Read the model definition and answer for the solid it produces. Units are mm, in the model's axes. A direction names the side the tool comes from. Coordinates: 2 decimals unless noted, no trailing zeros. Write each loop counter-clockwise with the first axis right and the second up, starting at its lowest first coordinate (ties: lowest second). Pieces come first, ordered by that corner, then holes. Notation, with made-up numbers: M -10,76 L 1,76 A23 cw 1,91 Z; hole C 47.25,15 d7. An arc over 180 degrees is marked long. Use a Markdown table: item, result. Add a question column.
from build123d import *

# Parameters (mm, degrees)
SKETCH1_W                                           = 75
SKETCH1_H                                           = 75
BOSS_EXTRUDE1_DEPTH                                 = 15
SKETCH2_R                                           = 22
BOSS_EXTRUDE2_DEPTH                                 = 5
CBORE_FOR_M5_HEX_SOCKET_HEAD_CAP_SCREW1_D           = 5.5
CBORE_FOR_M5_HEX_SOCKET_HEAD_CAP_SCREW1_CBORE_D     = 10
CBORE_FOR_M5_HEX_SOCKET_HEAD_CAP_SCREW1_CBORE_DEPTH = 5.4
CIRPATTERN1_COUNT                                   = 4
CHAMFER1_SIZE                                       = 6
SHELL1_START                                        = 3
SHELL1_OUTLINE_R                                    = 25
SHELL1_DEPTH                                        = 116.5
SHELL1_START_2                                      = -5
SHELL1_2_OUTLINE_R                                  = 14.94492882
SHELL1_2_DEPTH                                      = 206.012430393
SHELL1_3_OUTLINE_R                                  = 18.5
SHELL1_3_OUTLINE_R_2                                = 14.94492882
SHELL1_3_DEPTH                                      = 169.882661511
SHELL1_4_OUTLINE_R                                  = 25
SHELL1_4_DEPTH                                      = 9
SHELL1_5_OUTLINE_R                                  = 5.75
SHELL1_5_DEPTH                                      = 3.6
SHELL1_6_OUTLINE_R                                  = 19
SHELL1_6_OUTLINE_R_2                                = 18.5
SHELL1_6_DEPTH                                      = 8


with BuildPart() as part:
    # Sketch1 → Boss-Extrude1 (new body)
    with BuildSketch(Plane.XY):
        Rectangle(SKETCH1_W, SKETCH1_H)
    extrude(amount=BOSS_EXTRUDE1_DEPTH)

    # Sketch2 → Boss-Extrude2 (add)
    with BuildSketch(Plane(origin=(0, 0, 0), x_dir=(-1, 0, 0), z_dir=(0, 0, -1))):
        Circle(SKETCH2_R)
    extrude(amount=BOSS_EXTRUDE2_DEPTH)

    # Sketch3 → Revolve1 (revolve)
    with BuildSketch(Plane(origin=(0, 0, 0), x_dir=(0, 0, -1), z_dir=(1, 0, 0)), mode=Mode.PRIVATE) as revolve1_sk:
        Polygon((-15, 28), (-122.5, 28), (-122.5, 21.5), (-167.882661511, 21.5), (-167.882661511, 17.94492882), (-202.25507118, 17.94492882), (-207.2, 13), (-207.2, 0), (-15, 0), align=None)
    revolve(revolve1_sk.sketch.rotate(Axis((0, 0, 207.2), (0, 0, -1)), 90), axis=Axis((0, 0, 207.2), (0, 0, -1)))

    # CBORE for M5 Hex Socket Head Cap Screw1 (through all)
    with Locations(Plane.XY.offset(15)):
        with Locations((-27.5, 27.5)):
            cbore_for_m5_hex_socket_head_cap_screw1 = CounterBoreHole(CBORE_FOR_M5_HEX_SOCKET_HEAD_CAP_SCREW1_D / 2, CBORE_FOR_M5_HEX_SOCKET_HEAD_CAP_SCREW1_CBORE_D / 2, CBORE_FOR_M5_HEX_SOCKET_HEAD_CAP_SCREW1_CBORE_DEPTH)

    # CirPattern1: CBORE for M5 Hex Socket Head Cap Screw1 ×4 about axis
    cirpattern1_axis = Axis((0, 0, 0), (0, 0, 1))
    for i in range(1, CIRPATTERN1_COUNT):
        add(cbore_for_m5_hex_socket_head_cap_screw1.rotate(cirpattern1_axis, i * 360 / CIRPATTERN1_COUNT), mode=Mode.SUBTRACT)

    # Chamfer1
    chamfer1_edges = [part.edges().sort_by_distance(p)[0] for p in [
        (37.5, -37.5, 7.5),
        (-37.5, -37.5, 7.5),
        (-37.5, 37.5, 7.5),
        (37.5, 37.5, 7.5),
    ]]
    chamfer(chamfer1_edges, length=CHAMFER1_SIZE)

    # Shell1: read off the stored shape, not the designer's step
    # Shell1 outline → Shell1 (cut)
    with BuildSketch(Plane.XY.offset(SHELL1_START)):
        Circle(SHELL1_OUTLINE_R)
    extrude(amount=SHELL1_DEPTH, mode=Mode.SUBTRACT)

    # Shell1 2 outline → Shell1 2 (cut)
    with BuildSketch(Plane.XY.offset(SHELL1_START_2)):
        Circle(SHELL1_2_OUTLINE_R)
    extrude(amount=SHELL1_2_DEPTH, mode=Mode.SUBTRACT)

    # Shell1 3 outline → Shell1 3 (cut)
    with BuildSketch(Plane.XY.offset(SHELL1_START_2)):
        Circle(SHELL1_3_OUTLINE_R)
        Circle(SHELL1_3_OUTLINE_R_2, mode=Mode.SUBTRACT)
    extrude(amount=SHELL1_3_DEPTH, mode=Mode.SUBTRACT)

    # Shell1 4 outline → Shell1 4 (cut)
    with BuildSketch(Plane.XY.offset(SHELL1_START)):
        with BuildLine():
            Line((-34.5, 23.627016654), (-34.5, -23.627016654))
            ThreePointArc((-34.5, -23.627016654), (-21.843145751, -21.843145751), (-23.627016654, -34.5))
            Line((-23.627016654, -34.5), (23.627016654, -34.5))
            ThreePointArc((23.627016654, -34.5), (21.843145751, -21.843145751), (34.5, -23.627016654))
            Line((34.5, -23.627016654), (34.5, 23.627016654))
            ThreePointArc((34.5, 23.627016654), (21.843145751, 21.843145751), (23.627016654, 34.5))
            Line((23.627016654, 34.5), (-23.627016654, 34.5))
            ThreePointArc((-23.627016654, 34.5), (-21.843145751, 21.843145751), (-34.5, 23.627016654))
        make_face()
        Circle(SHELL1_4_OUTLINE_R, mode=Mode.SUBTRACT)
    extrude(amount=SHELL1_4_DEPTH, mode=Mode.SUBTRACT)

    # Shell1 5 outline → Shell1 5 (cut)
    # profile 1 of 4: a face of its own
    with BuildSketch(Plane.XY.offset(SHELL1_START)):
        with BuildLine():
            Line((-34.5, -23.627016654), (-34.5, -30.257359313))
            Line((-34.5, -30.257359313), (-30.257359313, -34.5))
            Line((-30.257359313, -34.5), (-23.627016654, -34.5))
            ThreePointArc((-23.627016654, -34.5), (-21.843145751, -21.843145751), (-34.5, -23.627016654))
        make_face()
        with Locations((-27.5, -27.5)):
            Circle(SHELL1_5_OUTLINE_R, mode=Mode.SUBTRACT)
    # profile 2 of 4: a face of its own
    with BuildSketch(Plane.XY.offset(SHELL1_START)):
        with BuildLine():
            Line((-34.5, 30.257359313), (-34.5, 23.627016654))
            ThreePointArc((-34.5, 23.627016654), (-21.843145751, 21.843145751), (-23.627016654, 34.5))
            Line((-23.627016654, 34.5), (-30.257359313, 34.5))
            Line((-30.257359313, 34.5), (-34.5, 30.257359313))
        make_face()
        with Locations((-27.5, 27.5)):
            Circle(SHELL1_5_OUTLINE_R, mode=Mode.SUBTRACT)
    # profile 3 of 4: a face of its own
    with BuildSketch(Plane.XY.offset(SHELL1_START)):
        with BuildLine():
            ThreePointArc((34.5, -23.627016654), (21.843145751, -21.843145751), (23.627016654, -34.5))
            Line((23.627016654, -34.5), (30.257359313, -34.5))
            Line((30.257359313, -34.5), (34.5, -30.257359313))
            Line((34.5, -30.257359313), (34.5, -23.627016654))
        make_face()
        with Locations((27.5, -27.5)):
            Circle(SHELL1_5_OUTLINE_R, mode=Mode.SUBTRACT)
    # profile 4 of 4: a face of its own
    with BuildSketch(Plane.XY.offset(SHELL1_START)):
        with BuildLine():
            Line((30.257359313, 34.5), (23.627016654, 34.5))
            ThreePointArc((23.627016654, 34.5), (21.843145751, 21.843145751), (34.5, 23.627016654))
            Line((34.5, 23.627016654), (34.5, 30.257359313))
            Line((34.5, 30.257359313), (30.257359313, 34.5))
        make_face()
        with Locations((27.5, 27.5)):
            Circle(SHELL1_5_OUTLINE_R, mode=Mode.SUBTRACT)
    extrude(amount=SHELL1_5_DEPTH, mode=Mode.SUBTRACT)

    # Shell1 6 outline → Shell1 6 (cut)
    with BuildSketch(Plane.XY.offset(SHELL1_START_2)):
        Circle(SHELL1_6_OUTLINE_R)
        Circle(SHELL1_6_OUTLINE_R_2, mode=Mode.SUBTRACT)
    extrude(amount=SHELL1_6_DEPTH, mode=Mode.SUBTRACT)

    # Shell1 7 outline → Shell1 7 (revolve, cut)
    with BuildSketch(Plane.XZ):
        Polygon((0, 201.012430393), (14.94492882, 201.012430426), (8.757359313, 207.2), (0, 207.2), align=None)
    revolve(axis=Axis((0, 0, 0), (0, 0, 1)), mode=Mode.SUBTRACT)


solid = part.part
Item 1: Find section A-A on z = 94. Give the vertices of the cut face in (x, y), then the cut area to 3 significant figures.
Item 2: Determine the mould class of faces 1 (the flat face through (-3.1, 8.5, 207.2)), 2 (the cylindrical face through (-2.799, -21.317, 145.509)), 3 (the flat face through (2.4, -25.4, 12)) for opening direction Z: pulls with the +Z half, pulls with the -Z half, needs draft (parallel to the pull), parting line crosses it, or undercut.
Item 3: Consider probe 1 along X at (y, z) = (-27, 6); probe 2 along X at (y, z) = (-27.5, 13.65); probe 3 along Z at (x, y) = (-17.5, 28.5). Determine where each line is inside the solid, lowest interval first.
Item 4: For faces 4 (the flat face through (-25, -25, 9.6)), 5 (the cylindrical face through (30.153, -32.601, 4.775)), 6 (the flat face through (35, 34, 7)), determine the directions among +Z, -Z, +X, -X, +Y, -Y from which every point of the face is accessible in a straight line to the end or side of a thin tool.
Item 5: Each of these flat-tipped pins is pushed along its axis until it touches: pin 1 (3 mm diameter, centred on y = 25.5, z = 33.5, fed in from +X); pin 2 (6 mm diameter, centred on x = 27.5, y = 27.5, fed in from -Z); pin 3 (12 mm diameter, centred on x = -19.5, z = 141.5, fed in from +Y). Where does it stop, or does it pass through?
Item 6: Find section B-B on z = 150.5. Give the vertices of the cut face in (x, y).
Geometry says:
| question | item | result |
|---|---|---|
| 1 | outline | C 0,0 d56; hole C 0,0 d50 |
| 1 | area | 500 mm2 |
| 2 | face 1 | pulls with the +Z half |
| 2 | face 2 | needs draft |
| 2 | face 3 | undercut |
| 3 | probe 1 | x = -37.5 to -34.5, -33.23 to -30.2, -24.8 to -21.77, 21.77 to 24.8, 30.2 to 33.23, 34.5 to 37.5 |
| 3 | probe 2 | x = -37.5 to -32.5, -22.5 to 22.5, 32.5 to 37.5 |
| 3 | probe 3 | z = 0 to 3, 12 to 15 |
| 4 | face 4 | +Z |
| 4 | face 5 | none |
| 4 | face 6 | +Z, -Z, +X, +Y |
| 5 | pin 1 | stops at x = 14.42 |
| 5 | pin 2 | stops at z = 0 |
| 5 | pin 3 | stops at y = 16.73 |
| 6 | outline | C 0,0 d43; hole C 0,0 d37 |
